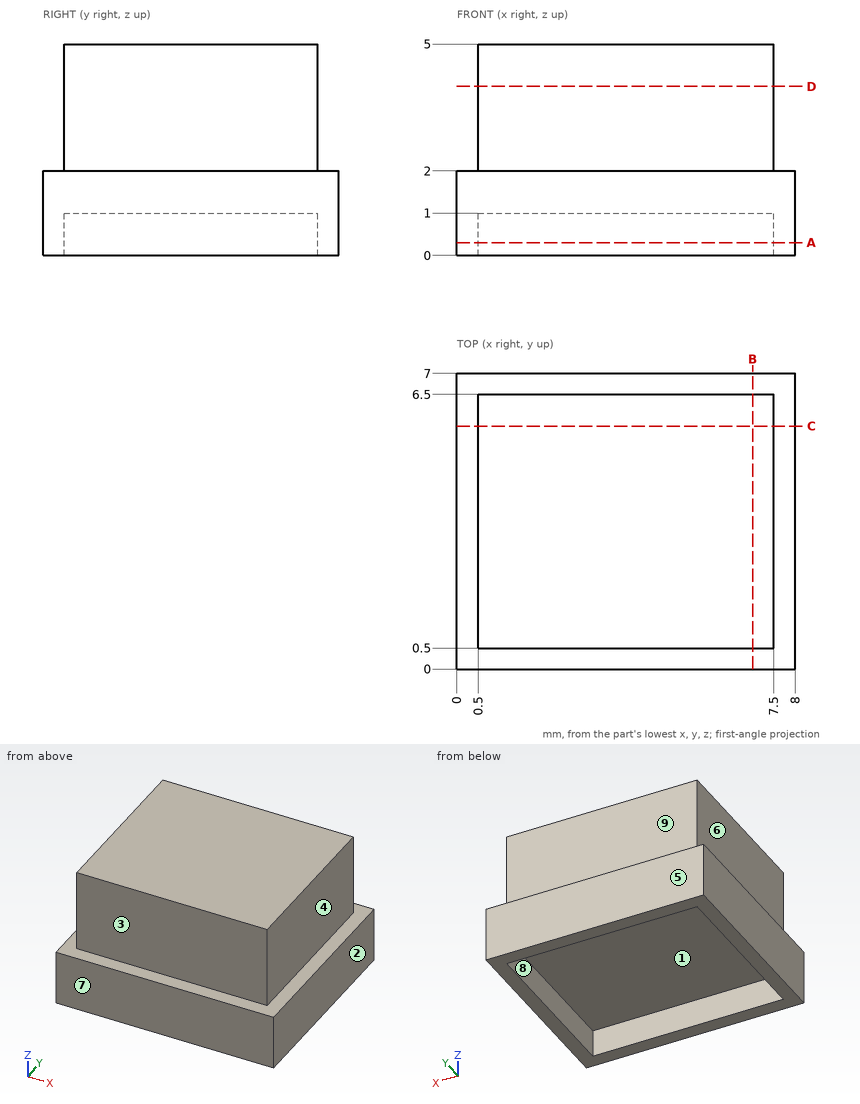
Verification items for this drawing (mm, ordinates from the low corner). A direction names the side the tool comes from. Give positions to 0.01 mm unless a question says otherwise; leave off trailing zeros. Write each loop counter-clockwise with the first axis right and the second up, starting at its lowest first coordinate (ties: lowest second). Pieces come first, ordered by that corner, then holes. Notation, with made-up numbers: (87, 55) -> (132, 55) arc R32 ccw to (132, 86) -> close; hole circle Ø3 at (69.25, -25). An arc over 180 degrees is marked (long way). Use one line per item in the form item = value.
Item 1: Depth check by flat-ended pin: pin 1 Ø3 at (x, y) = (4, 3) entering from -Z; pin 2 Ø0.9 at (x, z) = (4, 4) entering from -Y; pin 3 Ø2.5 at (x, z) = (4, 4) entering from +Y. Enter the tip coordinate at first touch or a pass-through.
Results list:
pin_1 = 1
pin_2 = 0.5
pin_3 = 6.5
Item 2: Scan lines: line 1 (Y direction, x = 6.5, z = 0.55); line 2 (X direction, y = 6, z = 0.5); line 3 (Y direction, x = 2.25, z = 3.4). Record each from-to range of solid material in increasing order.
Results list:
line_1 = 0 to 0.5, 6.5 to 7
line_2 = 0 to 0.5, 7.5 to 8
line_3 = 0.5 to 6.5
Item 3: Sectioned sample at D-D on z = 4. Enter the section's corners in (x, y).
Results list:
outline = (0.5, 0.5) -> (7.5, 0.5) -> (7.5, 6.5) -> (0.5, 6.5) -> close
Item 4: Sectioned sample at C-C on y = 5.75. Enter the section's corners in (x, z), plus the area to 3 significant figures.
Results list:
outline = (0, 0) -> (0.5, 0) -> (0.5, 1) -> (7.5, 1) -> (7.5, 0) -> (8, 0) -> (8, 2) -> (7.5, 2) -> (7.5, 5) -> (0.5, 5) -> (0.5, 2) -> (0, 2) -> close
area = 30.0 mm2
Item 5: Sectioned sample at A-A on z = 0.3. Enter the section's corners in (x, y).
Results list:
outline = (0, 0) -> (8, 0) -> (8, 7) -> (0, 7) -> close; hole (0.5, 0.5) -> (7.5, 0.5) -> (7.5, 6.5) -> (0.5, 6.5) -> close
Item 6: Mould release check, pull along Y, two halves, no side actions. Record for the marked faces 6, 7, 8 and 9: released by +Y, released by -Y, zero draft, split by the parting line, or undercut.
Results list:
face_6 = zero draft
face_7 = released by -Y
face_8 = undercut
face_9 = released by +Y
Item 7: Access from +Z, -Z, +X, -X, +Y, -Y to the whole of each face (thin tool, end or side, straight path). Record for the marked faces 1, 2, 3, 4 and 5.
Results list:
face_1 = -Z
face_2 = +Z, -Z, +X, +Y, -Y
face_3 = +Z, +X, -X, -Y
face_4 = +Z, +X, +Y, -Y
face_5 = +Z, -Z, +X, -X, +Y
Item 8: Sectioned sample at B-B on x = 7. Enter the section's corners in (y, z).
Results list:
outline = (0, 0) -> (0.5, 0) -> (0.5, 1) -> (6.5, 1) -> (6.5, 0) -> (7, 0) -> (7, 2) -> (6.5, 2) -> (6.5, 5) -> (0.5, 5) -> (0.5, 2) -> (0, 2) -> close
